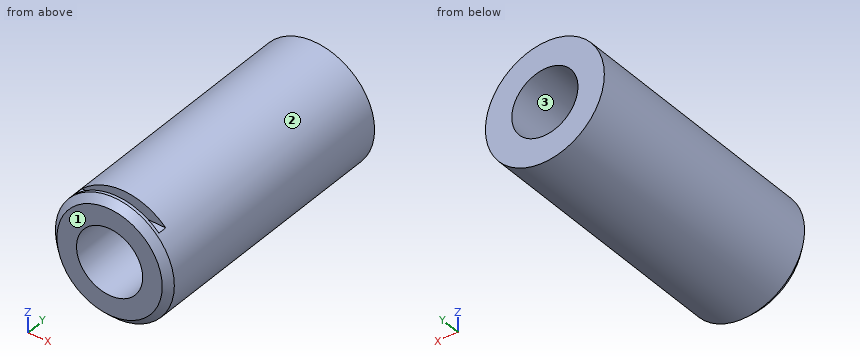
from build123d import *

# Parameters (mm, degrees)
F0_R     = 44.30014
F0_R_2   = 24.638
F1_DEPTH = 197.612
F3_W     = 88.9
F3_H     = 6.477
F4_DEPTH = 12.827
F5_SIZE  = 5.08


with BuildPart() as f1:
    # F0 (on Front) → F1 (new body)
    with BuildSketch(Plane.XZ):
        Circle(F0_R)
        Circle(F0_R_2, mode=Mode.SUBTRACT)
    extrude(amount=F1_DEPTH)

    # F3 (on offset) → F4 (cut)
    with BuildSketch(Plane.XY.offset(44.30014)):
        with Locations((0, -187.1345)):
            Rectangle(F3_W, F3_H)
    extrude(amount=-F4_DEPTH, mode=Mode.SUBTRACT)

    # F5
    f5_edges = [f1.edges().sort_by_distance(p)[0] for p in [
        (-44.30014, -197.612, 0),
    ]]
    chamfer(f5_edges, length=F5_SIZE)


solid = f1.part
Source: CAD feature listing. Evaluate the final solid. Frame: model axes, mm. Face numbers are marked on the shaded views. Give positions to 0.01 mm unless a question says otherwise; leave off trailing zeros. Write each loop counter-clockwise with the first axis right and the second up, starting at its lowest first coordinate (ties: lowest second). Pieces come first, ordered by that corner, then holes. Notation, with made-up numbers: (-4, -27) - (8, -27) arc R23 cw to (8, 11) - close; hole circle Ø1 at (47.25, -23). An arc over 180 degrees is marked (long way). Write item = value, one per line. Start each with the question number.
Q1. Draft query along X for the marked faces 1, 2 and 3. Return one class per face: +X half, -X half, draft (parallel to the pull), parting line (faces both ways), or undercut.
Q2. Pin query (flat end, axial travel): pin 1 Ø3 at (y, z) = (-25, -23) entering from +X; pin 2 Ø7 at (x, y) = (0, -186) entering from +Z; pin 3 Ø2 at (y, z) = (-150.5, -2) entering from -X. Return the tip coordinate at first contact, or that it passes through.
Q3. Cut plane C-C, the plane y = -33. Return loops of the section in (x, z).
Q4. Cut plane B-B, the plane z = 0. Return loops of the section in (x, y).
Q5. Cut plane A-A, the plane x = 0. Return loops of the section in (y, z).
Q6. Material intervals for probe 1 along Z at (x, y) = (0, -131.5); probe 2 along X at (y, z) = (-188, 1); probe 3 along Z at (x, y) = (-31.5, -112.5), sorted ascending.
Computed values:
q1.face_1 = draft
q1.face_2 = parting line
q1.face_3 = undercut
q2.pin_1 = 38.73
q2.pin_2 = 44.3
q2.pin_3 = -44.29
q3.outline = circle Ø88.6 at (0, 0); hole circle Ø49.28 at (0, 0)
q4.outline = (-44.3, -192.53) - (-39.22, -197.61) - (-24.64, -197.61) - (-24.64, 0) - (-44.3, 0) - close; (24.64, -197.61) - (39.22, -197.61) - (44.3, -192.53) - (44.3, 0) - (24.64, 0) - close
q5.outline = (-197.61, -39.22) - (-192.53, -44.3) - (0, -44.3) - (0, -24.64) - (-197.61, -24.64) - close; (-197.61, 24.64) - (0, 24.64) - (0, 44.3) - (-183.9, 44.3) - (-183.9, 31.47) - (-190.37, 31.47) - (-190.37, 44.3) - (-192.53, 44.3) - (-197.61, 39.22) - close
q6.probe_1 = -44.3 to -24.64, 24.64 to 44.3
q6.probe_2 = -44.29 to -24.62, 24.62 to 44.29
q6.probe_3 = -31.15 to 31.15
